Here's how the part is built. I have some questions about the finished solid (model axes, mm). Give positions to 0.01 mm unless a question says otherwise; leave off trailing zeros. Loops run counter-clockwise (first coordinate to the right, second up) from the corner with the lowest first, then second, coordinate; pieces in that order, holes last.
Q1. I need wall thicknesses on line 1 (Y direction, x = 116.4, z = 1.75); line 2 (Y direction, x = 188.4, z = 4.5); line 3 (X direction, y = 92.5, z = 4.25). Which ranges of each line are inside material? Lowest first, please.
Q2. If we section it at C-C (z = 1): Give the number of separate pieces and of enclosed holes in the cut face, plus the area to 3 significant figures.
Q3. If we section it at B-B (y = 107): Please give me the cut outline in (x, z).
Q4. If we section it at D-D (x = 106.5): Please give me the cut outline in (y, z).
Q5. We'd pull the mould along Y, two halves only. Please class faces 1 (the face through (406.892, 59.654, 3.131)), 2 (the face through (252.255, 126.567, 3.131)), 3 (the face through (264, 60, 6.35)): +Y half, -Y half, draft (parallel to the pull), parting line (faces both ways), or undercut.
Q6. Will these pins go through, and if not, where does the flat tip stop? P1, Ø1.8, axis at x = 116.4, y = 38.3, coming from the +Z side; P2, Ø3, axis at x = 402.5, z = 3, coming from the +Y side; P3, Ø1.5, axis at x = 343, z = 4, coming from the +Y side; P4, Ø1, axis at x = 259, z = 3.5, coming from the +Y side.
Q7. If we section it at A-A (x = 274): Please give me the cut outline in (y, z).
from build123d import *

# Parameters (mm, degrees)
SKETCH2_R           = 11
SKETCH2_R_2         = 1.5
SKETCH2_W           = 21
SKETCH2_H           = 13
BOSS_EXTRUDE1_DEPTH = 6.35


with BuildPart() as part:
    # Sketch2 → Boss-Extrude1 (new body)
    with BuildSketch(Plane.XY):
        Polygon((0, 152.4), (511.673882957, 100), (513.77689344, 120.535411062), (521.673882957, 119.726688428), (521.673882957, 101.6), (515.323882957, 101.6), (515.323882957, 50.8), (521.673882957, 50.8), (521.673882957, 0), (508, 0), (508, 6.35), (457.2, 6.35), (457.2, 0), (406.4, 0), (406.4, 6.35), (355.6, 6.35), (355.6, 0), (304.8, 0), (304.8, 6.35), (254, 6.35), (254, 0), (203.2, 0), (203.2, 6.35), (152.4, 6.35), (152.4, 0), (101.6, 0), (101.6, 6.35), (50.8, 6.35), (50.8, 0), (0, 0), (0, 50.8), (6.35, 50.8), (6.35, 101.6), (0, 101.6), align=None)
        with Locations((396.4, 56.35)):
            Circle(SKETCH2_R, mode=Mode.SUBTRACT)
        with Locations((116.4, 63.3)):
            Circle(SKETCH2_R_2, mode=Mode.SUBTRACT)
        with Locations((188.4, 63.3)):
            Circle(SKETCH2_R_2, mode=Mode.SUBTRACT)
        with Locations((188.4, 38.3)):
            Circle(SKETCH2_R_2, mode=Mode.SUBTRACT)
        with Locations((116.4, 38.3)):
            Circle(SKETCH2_R_2, mode=Mode.SUBTRACT)
        Polygon((180.4, 58.3), (191.4, 58.3), (191.4, 43.3), (180.4, 43.3), (180.4, 35.3), (124.4, 35.3), (124.4, 43.3), (113.4, 43.3), (113.4, 58.3), (124.4, 58.3), (124.4, 66.3), (180.4, 66.3), align=None, mode=Mode.SUBTRACT)
        with Locations((457.2, 36.35)):
            Rectangle(SKETCH2_W, SKETCH2_H, mode=Mode.SUBTRACT)
        with BuildLine():
            Line((249.0403247, 35.3), (249.0403247, 70.684208401))
            ThreePointArc((249.0403247, 70.684208401), (254, 75.643883701), (258.9596753, 70.684208401))
            Line((258.9596753, 70.684208401), (258.9596753, 35.3))
            ThreePointArc((258.9596753, 35.3), (254, 30.3403247), (249.0403247, 35.3))
        make_face(mode=Mode.SUBTRACT)
        with BuildLine():
            Line((269.0403247, 35.3), (269.0403247, 70.684208401))
            ThreePointArc((269.0403247, 70.684208401), (274, 75.643883701), (278.9596753, 70.684208401))
            Line((278.9596753, 70.684208401), (278.9596753, 35.3))
            ThreePointArc((278.9596753, 35.3), (274, 30.3403247), (269.0403247, 35.3))
        make_face(mode=Mode.SUBTRACT)
        with BuildLine():
            Line((289.0403247, 35.3), (289.0403247, 70.684208401))
            ThreePointArc((289.0403247, 70.684208401), (294, 75.643883701), (298.9596753, 70.684208401))
            Line((298.9596753, 70.684208401), (298.9596753, 35.3))
            ThreePointArc((298.9596753, 35.3), (294, 30.3403247), (289.0403247, 35.3))
        make_face(mode=Mode.SUBTRACT)
        with BuildLine():
            Line((309.0403247, 35.3), (309.0403247, 70.684208401))
            ThreePointArc((309.0403247, 70.684208401), (314, 75.643883701), (318.9596753, 70.684208401))
            Line((318.9596753, 70.684208401), (318.9596753, 35.3))
            ThreePointArc((318.9596753, 35.3), (314, 30.3403247), (309.0403247, 35.3))
        make_face(mode=Mode.SUBTRACT)
        with BuildLine():
            Line((329.0403247, 35.3), (329.0403247, 70.684208401))
            ThreePointArc((329.0403247, 70.684208401), (334, 75.643883701), (338.9596753, 70.684208401))
            Line((338.9596753, 70.684208401), (338.9596753, 35.3))
            ThreePointArc((338.9596753, 35.3), (334, 30.3403247), (329.0403247, 35.3))
        make_face(mode=Mode.SUBTRACT)
    extrude(amount=BOSS_EXTRUDE1_DEPTH)


solid = part.part
Check sheet entries:
1. line 1: y = 0 to 36.8, 39.8 to 43.3, 58.3 to 61.8, 64.8 to 140.48
1. line 2: y = 6.35 to 36.8, 39.8 to 43.3, 58.3 to 61.8, 64.8 to 133.11
1. line 3: x = 6.35 to 515.32
2. separate pieces: 1
2. enclosed holes: 12
2. area: 58,600 mm2
3. outline: (0, 0) - (443.32, 0) - (443.32, 6.35) - (0, 6.35) - close; (512.39, 0) - (521.67, 0) - (521.67, 6.35) - (512.39, 6.35) - close
4. outline: (0, 0) - (141.49, 0) - (141.49, 6.35) - (0, 6.35) - close
5. face 1: undercut
5. face 2: +Y half
5. face 3: draft
6. P1: passes through
6. P2: stops at y = 111.33
6. P3: stops at y = 117.35
6. P4: stops at y = 125.93
7. outline: (6.35, 0) - (30.34, 0) - (30.34, 6.35) - (6.35, 6.35) - close; (75.64, 0) - (124.34, 0) - (124.34, 6.35) - (75.64, 6.35) - close
